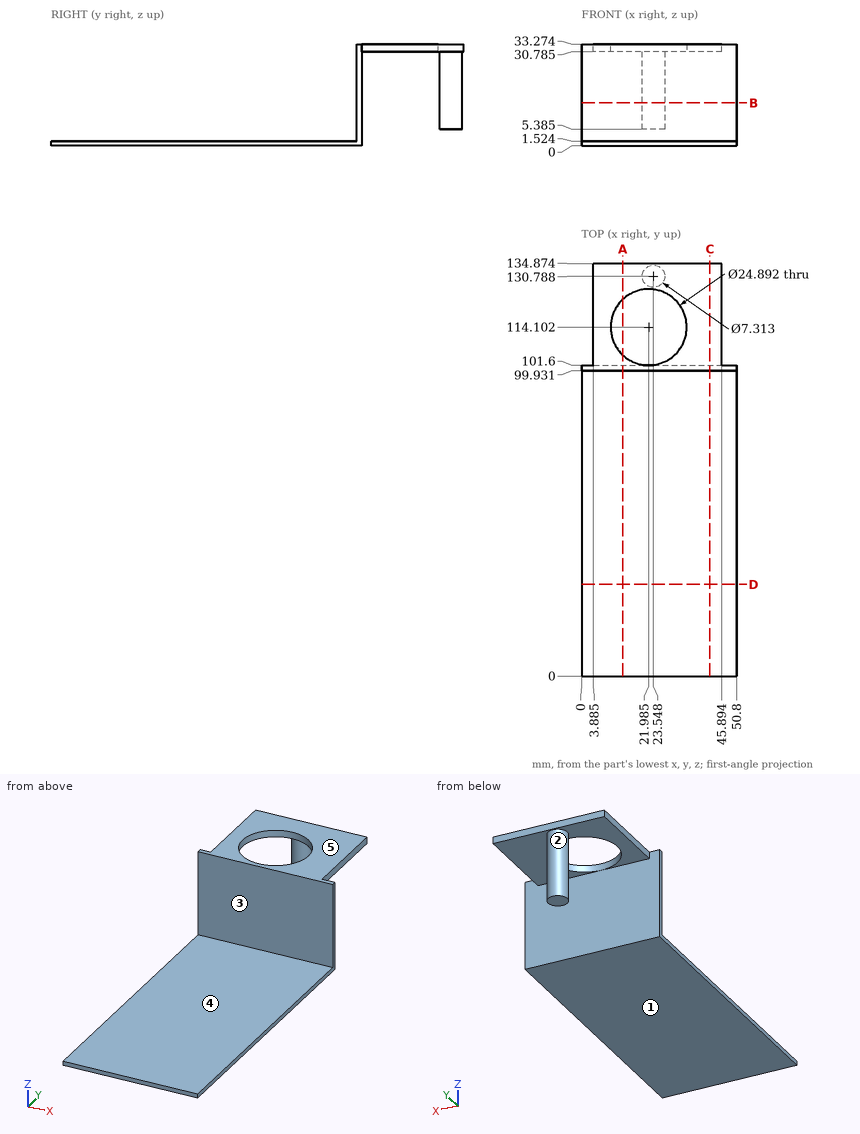
The drawing under review shows one solid part. Ordinate dimensions are in mm from its lowest x, y, z. A direction names the side the tool comes from. Round coordinates to 2 decimals unless told otherwise and drop trailing zeros. Write each loop counter-clockwise with the first axis right and the second up, starting at its lowest first coordinate (ties: lowest second). Pieces come first, ordered by that corner, then holes. Notation, with made-up numbers: (60, -11.5) - (69, -11.5) arc R27 cw to (69, 22.5) - close; hole circle Ø6 at (59, -23.75). An arc over 180 degrees is marked (long way). Use one line per item in the form item = value.
Q1. Consider section D-D (y = 30). State the section outline as (x, z) points.
Answer key:
outline = (0, 0) - (50.8, 0) - (50.8, 1.52) - (0, 1.52) - close
Q2. Insertion check: pin 1 Ø22.5 at (x, y) = (21.99, 114.1) entering from -Z; pin 2 Ø1.2 at (y, z) = (122, 32) entering from +X; pin 3 Ø10 at (x, y) = (35, 108) entering from -Z (1 decimal); pin 4 Ø1.5 at (x, z) = (28.5, 29) entering from -Y. Each pin has a flat end and moves straight along its axis. Give the tip position at first contact, or say it passes through.
Answer key:
pin_1 = through
pin_2 = 45.89
pin_3 = 30.8
pin_4 = 99.93
Q3. Consider section C-C (x = 42). State the section outline as (y, z) points (1 decimal).
Answer key:
outline = (0, 0) - (101.6, 0) - (101.6, 30.8) - (134.9, 30.8) - (134.9, 33.3) - (99.9, 33.3) - (99.9, 1.5) - (0, 1.5) - close
Q4. Tool access review of the marked faces 4 and 5: name each direction out of +Z, -Z, +X, -X, +Y, -Y from which nothing blocks a thin tool from reaching the whole face with its end or side.
Answer key:
face_4 = +Z, +X, -X, -Y
face_5 = +Z, +X, -X, +Y, -Y
Q5. Draft analysis for pull direction Y (two halves, no side actions). For the marked faces 1, 2 and 3, state which applies: +Y half, -Y half, draft (parallel to the pull), parting line (faces both ways), or undercut.
Answer key:
face_1 = draft
face_2 = undercut
face_3 = -Y half
Q6. Consider section A-A (x = 13.5). State the section outline as (y, z) points (1 decimal).
Answer key:
outline = (0, 0) - (101.6, 0) - (101.6, 30.8) - (105, 30.8) - (105, 33.3) - (99.9, 33.3) - (99.9, 1.5) - (0, 1.5) - close; (123.2, 30.8) - (134.9, 30.8) - (134.9, 33.3) - (123.2, 33.3) - close
Q7. For line 1 (Y direction, x = 3.5, z = 11); line 2 (Z direction, x = 47, y = 49); line 3 (Z direction, x = 7.5, y = 108.5) (1 decimal), list the stretches that pass through material, from the lowest coordinate up. Write a range as [from, to].
Answer key:
line_1 = [99.93, 101.6]
line_2 = [0, 1.52]
line_3 = [30.8, 33.3]
Q8. Consider section B-B (z = 14). State the section outline as (x, y) points (1 decimal).
Answer key:
outline = (0, 99.9) - (50.8, 99.9) - (50.8, 101.6) - (0, 101.6) - close; circle Ø7.3 at (23.5, 130.8)
